```python
from build123d import *

# Parameters (mm, degrees)
SKETCH1_R           = 13.1699
BOSS_EXTRUDE1_DEPTH = 1.27
SKETCH2_R           = 13.1699
SKETCH2_R_2         = 12.0523
BOSS_EXTRUDE2_DEPTH = 0.762
SKETCH3_R           = 1.4351
BOSS_EXTRUDE3_DEPTH = 11.5443
SKETCH6_W           = 7.112
SKETCH6_H           = 5.842
BOSS_EXTRUDE4_DEPTH = 0.4318
SKETCH7_W           = 7.112
SKETCH7_H           = 5.842
BOSS_EXTRUDE5_DEPTH = 0.4318
SKETCH4_R           = 0.7874
CUT_EXTRUDE1_DEPTH  = 11.5443


with BuildPart() as part:
    # Sketch1 → Boss-Extrude1 (new body)
    with BuildSketch(Plane(origin=(0, 0, 0), x_dir=(1, 0, 0), z_dir=(0, 1, 0))):
        Circle(SKETCH1_R)
    extrude(amount=BOSS_EXTRUDE1_DEPTH)

    # Sketch2 → Boss-Extrude2 (add)
    with BuildSketch(Plane(origin=(0, 1.27, 0), x_dir=(1, 0, 0), z_dir=(0, 1, 0))):
        Circle(SKETCH2_R)
        Circle(SKETCH2_R_2, mode=Mode.SUBTRACT)
    extrude(amount=BOSS_EXTRUDE2_DEPTH)

    # Sketch3 → Boss-Extrude3 (add)
    with BuildSketch(Plane(origin=(0, 1.27, 0), x_dir=(1, 0, 0), z_dir=(0, 1, 0))):
        Circle(SKETCH3_R)
    extrude(amount=BOSS_EXTRUDE3_DEPTH)

    # Sketch6 → Boss-Extrude4 (add, symmetric)
    with BuildSketch(Plane.XY):
        with Locations((0, 2.921)):
            Rectangle(SKETCH6_W, SKETCH6_H)
    extrude(amount=BOSS_EXTRUDE4_DEPTH, both=True)

    # Sketch7 → Boss-Extrude5 (add, symmetric)
    with BuildSketch(Plane(origin=(0, 0, 0), x_dir=(0, 0, -1), z_dir=(1, 0, 0))):
        with Locations((0, 2.921)):
            Rectangle(SKETCH7_W, SKETCH7_H)
    extrude(amount=BOSS_EXTRUDE5_DEPTH, both=True)

    # Sketch4 → Cut-Extrude1 (cut)
    with BuildSketch(Plane(origin=(0, 12.8143, 0), x_dir=(1, 0, 0), z_dir=(0, 1, 0))):
        Circle(SKETCH4_R)
    extrude(amount=-CUT_EXTRUDE1_DEPTH, mode=Mode.SUBTRACT)


solid = part.part
```
Part model, mm, in its own coordinate system. A direction names the side the tool comes from. Round coordinates to 2 decimals unless told otherwise and drop trailing zeros. Write each loop counter-clockwise with the first axis right and the second up, starting at its lowest first coordinate (ties: lowest second). Pieces come first, ordered by that corner, then holes.
Item 1: Cut at A-A, the plane x = 0. Give the cut face in (y, z), plus the area to 3 significant figures.
Results:
outline: (0, -13.17) - (2.03, -13.17) - (2.03, -12.05) - (1.27, -12.05) - (1.27, -3.56) - (5.84, -3.56) - (5.84, -1.44) - (12.81, -1.44) - (12.81, -0.79) - (1.27, -0.79) - (1.27, 0.79) - (12.81, 0.79) - (12.81, 1.44) - (5.84, 1.44) - (5.84, 3.56) - (1.27, 3.56) - (1.27, 12.05) - (2.03, 12.05) - (2.03, 13.17) - (0, 13.17) - close
area: 69.5 mm2
Item 2: Cut at D-D, the plane x = -10.25. Give the cut face in (y, z).
Results:
outline: (0, -8.27) - (2.03, -8.27) - (2.03, -6.34) - (1.27, -6.34) - (1.27, 6.34) - (2.03, 6.34) - (2.03, 8.27) - (0, 8.27) - close
Item 3: Which spindle directions (+Z, -Z, +X, -X, +Y, -Y) get a long thin tool onto all of the face, cutting with end or side? Do faces 1 (the flat face through (0, 0, 0)), 2 (the flat face through (0, 1.27, 0)). Say none if no direction does.
Results:
face 1: +Z, -Z, +X, -X, -Y
face 2: +Y
Item 4: Two-plate mould, pull along X, no slides. Class faces 3 (the flat face through (3, 1.27, 3)), 4 (the flat face through (0, 12.814, 1)), 5 (the cylindrical face through (-10.451, 1.002, 8.014)), 6 (the cylindrical face through (-1.57, 1.65, -11.95)): +X half, -X half, draft (parallel to the pull), parting line (faces both ways), or undercut.
Results:
face 3: undercut
face 4: draft
face 5: parting line
face 6: undercut
Item 5: Probe L1, parallel to Z at x = 0, y = 1.7; L2, parallel to Y at x = 4.25, z = -5.5. List the from-to ranges inside material, lowest first.
Results:
L1: z = -13.17 to -12.05, -3.56 to -0.79, 0.79 to 3.56, 12.05 to 13.17
L2: y = 0 to 1.27
Item 6: Drop flat-ended pins along their axis: pin 1 Ø1.1 at (x, y) = (2, 4) entering from -Z; pin 2 Ø1.7 at (y, z) = (4, -3) entering from +X; pin 3 Ø3 at (x, z) = (0.5, -5) entering from +Y; pin 4 Ø3 at (x, y) = (-4, 10) entering from +Z. Give the stop position or say it passes through.
Results:
pin 1: stops at z = -0.43
pin 2: stops at x = 0.43
pin 3: stops at y = 5.84
pin 4: passes through
Item 7: Cut at B-B, the plane y = 3.5. Give the cut face in (x, z), plus the area to 3 significant figures.
Results:
outline: (-3.56, -0.43) - (-1.37, -0.43) arc R1.44 ccw to (-0.43, -1.37) - (-0.43, -3.56) - (0.43, -3.56) - (0.43, -1.37) arc R1.44 ccw to (1.37, -0.43) - (3.56, -0.43) - (3.56, 0.43) - (1.37, 0.43) arc R1.44 ccw to (0.43, 1.37) - (0.43, 3.56) - (-0.43, 3.56) - (-0.43, 1.37) arc R1.44 ccw to (-1.37, 0.43) - (-3.56, 0.43) - close; hole circle Ø1.57 at (0, 0)
area: 11.9 mm2
Item 8: Cut at C-C, the plane z = -8.75. Give the cut face in (x, y).
Results:
outline: (-9.84, 0) - (9.84, 0) - (9.84, 2.03) - (8.29, 2.03) - (8.29, 1.27) - (-8.29, 1.27) - (-8.29, 2.03) - (-9.84, 2.03) - close
